from build123d import *

# Parameters (mm, degrees)
PAD004_DEPTH   = 0.2
SKETCH003_R    = 1.25
PAD005_DEPTH   = 30
PRISM_DEPTH    = 3
PRISM001_DEPTH = 3


with BuildPart() as part:
    # Sketch008 → Pad004 (new body)
    with BuildSketch(Plane.XY.offset(-1)):
        with BuildLine():
            ThreePointArc((-1.5, 0), (0, -1.5), (1.5, 0))
            Line((1.5, 12.73), (1.5, 0))
            ThreePointArc((1.5, 12.73), (0, 14.23), (-1.5, 12.73))
            Line((-1.5, 12.73), (-1.5, 0))
        make_face()
    extrude(amount=-PAD004_DEPTH)

    # Sketch003 → Pad005 (join)
    with BuildSketch(Plane.XY.offset(-1)):
        Circle(SKETCH003_R)
        with Locations((0, 12.73)):
            Circle(SKETCH003_R)
    extrude(amount=PAD005_DEPTH)

    # Prism → Prism (join)
    with BuildSketch(Plane(origin=(0, 0, 0), x_dir=(0, 1, 0), z_dir=(0, 0, 1))):
        Polygon((3.35, 0), (1.675, 2.901185), (-1.675, 2.901185), (-3.35, 0), (-1.675, -2.901185), (1.675, -2.901185), align=None)
    extrude(amount=PRISM_DEPTH)

    # Prism001 → Prism001 (join)
    with BuildSketch(Plane(origin=(0, 12.73, 0), x_dir=(0, 1, 0), z_dir=(0, 0, 1))):
        Polygon((3.35, 0), (1.675, 2.901185), (-1.675, 2.901185), (-3.35, 0), (-1.675, -2.901185), (1.675, -2.901185), align=None)
    extrude(amount=PRISM001_DEPTH)


solid = part.part
The listing builds one solid part. Answer for the finished solid, in the listing's coordinates (mm). A direction names the side the tool comes from. Coordinates: 2 decimals unless noted, no trailing zeros. Write each loop counter-clockwise with the first axis right and the second up, starting at its lowest first coordinate (ties: lowest second). Pieces come first, ordered by that corner, then holes. Notation, with made-up numbers: M -8,6 L 15,6 A22 cw 15,36 Z; hole C 57,65.25 d5. An arc over 180 degrees is marked long. Use one line per item in the form item = value.
Item 1: Find section A-A, the plane x = 2.45. Give the vertices of the cut face in (y, z).
Model answer:
outline = M -1.94,0 L 1.94,0 L 1.94,3 L -1.94,3 Z; M 10.79,0 L 14.67,0 L 14.67,3 L 10.79,3 Z
Item 2: Given P1, Ø1, axis at x = 2.5, z = 18.5, coming from the +Y side; P2, Ø8, axis at y = 0, z = 24.5, coming from the +X side; P3, Ø0.9, axis at x = 0, y = 4, coming from the +Z side; P4, Ø4, axis at y = 10, z = 23, coming from the +X side, each flat-ended and moving along its own axis, determine where each tip first touches the part or whether it passes through.
Model answer:
P1 = through
P2 = 1.25
P3 = -1
P4 = 1.01
Item 3: For faces 1 (the face through (1.43, 10.206, 1.479)), 2 (the face through (-1.47, 10.23, 1.48)), 3 (the face through (-0.27, -1.22, -0.51)), 4 (the face through (0, 14.2, 3)), determine the directions among +Z, -Z, +X, -X, +Y, -Y from which every point of the face is accessible in a straight line to the end or side of a thin tool.
Model answer:
face_1 = +Z, +X
face_2 = +Z, -X
face_3 = none
face_4 = +Z
Item 4: Find section B-B, the plane z = 25. Give the vertices of the cut face in (x, y), plus the area to 3 significant figures.
Model answer:
outline = C 0,0 d2.5; C 0,12.73 d2.5
area = 9.82 mm2
Item 5: The mould has two halves that part along Y. Classify faces 5 (the face through (1.47, 15.23, 1.48)), 6 (the face through (1.47, 2.5, 1.48)), 7 (the face through (0, 13, 29)): released by +Y, released by -Y, zero draft, split by the parting line, or undercut.
Model answer:
face_5 = released by +Y
face_6 = undercut
face_7 = zero draft
Item 6: Find section C-C, the plane x = -0.5. Give the vertices of the cut face in (y, z), plus the area to 3 significant figures.
Model answer:
outline = M -3.06,0 L -1.15,0 L -1.15,-1 L -1.41,-1 L -1.41,-1.2 L 14.14,-1.2 L 14.14,-1 L 13.88,-1 L 13.88,0 L 15.79,0 L 15.79,3 L 13.88,3 L 13.88,29 L 11.58,29 L 11.58,3 L 9.67,3 L 9.67,0 L 11.58,0 L 11.58,-1 L 1.15,-1 L 1.15,0 L 3.06,0 L 3.06,3 L 1.15,3 L 1.15,29 L -1.15,29 L -1.15,3 L -3.06,3 Z
area = 164 mm2
Item 7: Find the intervals of material crossed by probe 1 along Z at (x, y) = (0.45, 1.25); probe 2 along Y at (x, z) = (-1.8, 2); probe 3 along Y at (x, z) = (0.65, 4), in increasing order.
Model answer:
probe_1 = -1.2 to -1, 0 to 3
probe_2 = -2.31 to 2.31, 10.42 to 15.04
probe_3 = -1.07 to 1.07, 11.66 to 13.8
Item 8: Find section D-D, the plane y = 7. Give the vertices of the cut face in (x, z).
Model answer:
outline = M -1.5,-1.2 L 1.5,-1.2 L 1.5,-1 L -1.5,-1 Z
